Part model, mm, in its own coordinate system. Face numbers are marked on the shaded views. A direction names the side the tool comes from. Round coordinates to 2 decimals unless told otherwise and drop trailing zeros. Order: outer loops, then holes, each group sorted by start corner. A loop starts at its lowest first (then second) coordinate and runs counter-clockwise, first axis right, second up. Notation, with made-up numbers: (75, 62) -> (115, 62) arc R19 cw to (115, 73) -> close; hole circle Ø1 at (6, 87.5). An arc over 180 degrees is marked (long way). Answer as a JSON object with one key per item and string values. Group by question number.
```python
from build123d import *

# Parameters (mm, degrees)
SKETCH_1_W           = 20
SKETCH_1_H           = 20
EXTRUDE_1_DEPTH      = 120
SKETCH_2_W           = 10
SKETCH_2_H           = 20
CUT_EXTRUDE_1_DEPTH  = 120
CUT_EXTRUDE_2_DEPTH  = 120
SKETCH_4_R           = 3
CUT_EXTRUDE_3_DEPTH  = 2
SKETCH_8_W           = 19.6
SKETCH_8_H           = 0.2
SKETCH_8_W_2         = 0.2
SKETCH_8_H_2         = 19.6
CUT_EXTRUDE_6_DEPTH  = 15
SKETCH_9_W           = 10
SKETCH_9_H           = 20
CUT_EXTRUDE_7_DEPTH  = 20
SKETCH_10_W          = 19.6
SKETCH_10_H          = 19.6
EXTRUDE_2_DEPTH      = 15
CUT_EXTRUDE_8_DEPTH  = 20
CUT_EXTRUDE_9_DEPTH  = 20
SKETCH_13_W          = 55
SKETCH_13_H          = 20
SKETCH_13_W_2        = 18.82824967
CUT_EXTRUDE_10_DEPTH = 20
SKETCH_14_W          = 100
SKETCH_14_H          = 55
EXTRUDE_5_DEPTH      = 5
SKETCH_17_W          = 2
SKETCH_17_H          = 55
CUT_EXTRUDE_12_DEPTH = 1000
EXTRUDE_6_DEPTH      = 94
SKETCH_19_W          = 3
SKETCH_19_H          = 55
EXTRUDE_7_DEPTH      = 100


with BuildPart() as part:
    # 草图1 → 凸台-拉伸1 (new body)
    with BuildSketch(Plane.XY):
        with Locations((10, 10)):
            Rectangle(SKETCH_1_W, SKETCH_1_H)
    extrude(amount=EXTRUDE_1_DEPTH)

    # 草图2 → 切除-拉伸1 (cut)
    with BuildSketch(Plane(origin=(0, 20, 0), x_dir=(1, 0, 0), z_dir=(0, 1, 0))):
        with Locations((15, -10)):
            Rectangle(SKETCH_2_W, SKETCH_2_H)
    extrude(amount=-CUT_EXTRUDE_1_DEPTH, mode=Mode.SUBTRACT)

    # 草图3 → 切除-拉伸2 (cut)
    with BuildSketch(Plane(origin=(10, 0, 0), x_dir=(0, 0, -1), z_dir=(1, 0, 0))):
        with BuildLine():
            ThreePointArc((-8.45, 10), (-9.40684068, 11.432013275), (-11.096015511, 11.096015511))
            Line((-11.096015511, 11.096015511), (-8.903984489, 8.903984489))
            ThreePointArc((-8.903984489, 8.903984489), (-8.567986725, 9.40684068), (-8.45, 10))
        make_face()
        with BuildLine():
            Line((-8.903984489, 8.903984489), (-11.096015511, 11.096015511))
            ThreePointArc((-11.096015511, 11.096015511), (-11.096015511, 8.903984489), (-8.903984489, 8.903984489))
        make_face()
    extrude(amount=-CUT_EXTRUDE_2_DEPTH, mode=Mode.SUBTRACT)

    # 草图4 → 切除-拉伸3 (cut)
    with BuildSketch(Plane.ZY):
        with Locations((10, 10)):
            Circle(SKETCH_4_R)
    extrude(amount=-CUT_EXTRUDE_3_DEPTH, mode=Mode.SUBTRACT)

    # 草图8 → 切除-拉伸6 (cut)
    with BuildSketch(Plane.XY.offset(120)):
        with Locations((10, 19.9)):
            Rectangle(SKETCH_8_W, SKETCH_8_H)
        with Locations((0.1, 19.9)):
            Rectangle(SKETCH_8_W_2, SKETCH_8_H)
        with Locations((0.1, 10)):
            Rectangle(SKETCH_8_W_2, SKETCH_8_H_2)
        with Locations((19.9, 10)):
            Rectangle(SKETCH_8_W_2, SKETCH_8_H_2)
        with Locations((19.9, 0.1)):
            Rectangle(SKETCH_8_W_2, SKETCH_8_H)
        with Locations((10, 0.1)):
            Rectangle(SKETCH_8_W, SKETCH_8_H)
        with Locations((0.1, 0.1)):
            Rectangle(SKETCH_8_W_2, SKETCH_8_H)
        with Locations((19.9, 19.9)):
            Rectangle(SKETCH_8_W_2, SKETCH_8_H)
    extrude(amount=-CUT_EXTRUDE_6_DEPTH, mode=Mode.SUBTRACT)

    # 草图9 → 切除-拉伸7 (cut)
    with BuildSketch(Plane(origin=(0, 20, 0), x_dir=(1, 0, 0), z_dir=(0, 1, 0))):
        Polygon((0, 0), (0, -45), (20, -45), (20, -20), (10, -20), (10, 0), align=None)
        with Locations((15, -10)):
            Rectangle(SKETCH_9_W, SKETCH_9_H)
    extrude(amount=-CUT_EXTRUDE_7_DEPTH, mode=Mode.SUBTRACT)

    # 草图10 → 凸台-拉伸2 (add)
    with BuildSketch(Plane(origin=(0, 0, 45), x_dir=(-1, 0, 0), z_dir=(0, 0, -1))):
        with Locations((-10, 10)):
            Rectangle(SKETCH_10_W, SKETCH_10_H)
    extrude(amount=EXTRUDE_2_DEPTH)

    # 草图11 → 切除-拉伸8 (cut)
    with BuildSketch(Plane(origin=(0, 19.8, 0), x_dir=(1, 0, 0), z_dir=(0, 1, 0))):
        with BuildLine():
            ThreePointArc((11.547573501, -112.5), (10.487812185, -111.029569439), (8.757681845, -111.569855559))
            Line((8.757681845, -111.569855559), (11.237465157, -113.430144441))
            ThreePointArc((11.237465157, -113.430144441), (11.468004062, -112.990238683), (11.547573501, -112.5))
        make_face()
        with BuildLine():
            Line((11.237465157, -113.430144441), (8.757681845, -111.569855559))
            ThreePointArc((8.757681845, -111.569855559), (9.06742906, -113.739891656), (11.237465157, -113.430144441))
        make_face()
    extrude(amount=-CUT_EXTRUDE_8_DEPTH, mode=Mode.SUBTRACT)

    # 草图12 → 切除-拉伸9 (cut)
    with BuildSketch(Plane(origin=(0, 19.8, 0), x_dir=(1, 0, 0), z_dir=(0, 1, 0))):
        with BuildLine():
            ThreePointArc((11.55, -37.5), (10.490153037, -36.029540888), (8.76, -36.57))
            Line((8.76, -36.57), (11.24, -38.43))
            ThreePointArc((11.24, -38.43), (11.470459112, -37.990153037), (11.55, -37.5))
        make_face()
        with BuildLine():
            Line((11.24, -38.43), (8.76, -36.57))
            ThreePointArc((8.76, -36.57), (9.07, -38.74), (11.24, -38.43))
        make_face()
    extrude(amount=-CUT_EXTRUDE_9_DEPTH, mode=Mode.SUBTRACT)

    # 草图13 → 切除-拉伸10 (cut)
    with BuildSketch(Plane.ZY):
        with Locations((77.5, 10)):
            Rectangle(SKETCH_13_W, SKETCH_13_H)
        with Locations((114.414124835, 10)):
            Rectangle(SKETCH_13_W_2, SKETCH_13_H)
    extrude(amount=-CUT_EXTRUDE_10_DEPTH, mode=Mode.SUBTRACT)

    # 草图14 → 凸台-拉伸5 (add)
    with BuildSketch(Plane.XY.offset(50)):
        with Locations((10, 17.5)):
            Rectangle(SKETCH_14_W, SKETCH_14_H)
    extrude(amount=-EXTRUDE_5_DEPTH)

    # 草图17 → 切除-拉伸12 (cut)
    with BuildSketch(Plane.ZY.offset(40)):
        with Locations((49, 17.5)):
            Rectangle(SKETCH_17_W, SKETCH_17_H)
    extrude(amount=-CUT_EXTRUDE_12_DEPTH, mode=Mode.SUBTRACT)

    # 草图18 → 凸台-拉伸6 (add)
    with BuildSketch(Plane.XY.offset(48)):
        Polygon((-40, -10), (60, -10), (60, 45), (57, 45), (57, -7), (-37, -7), (-37, 45), (-40, 45), align=None)
    extrude(amount=EXTRUDE_6_DEPTH)

    # 草图19 → 凸台-拉伸7 (add)
    with BuildSketch(Plane(origin=(60, 0, 0), x_dir=(0, 0, -1), z_dir=(1, 0, 0))):
        with Locations((-143.5, 17.5)):
            Rectangle(SKETCH_19_W, SKETCH_19_H)
    extrude(amount=-EXTRUDE_7_DEPTH)


solid = part.part
```
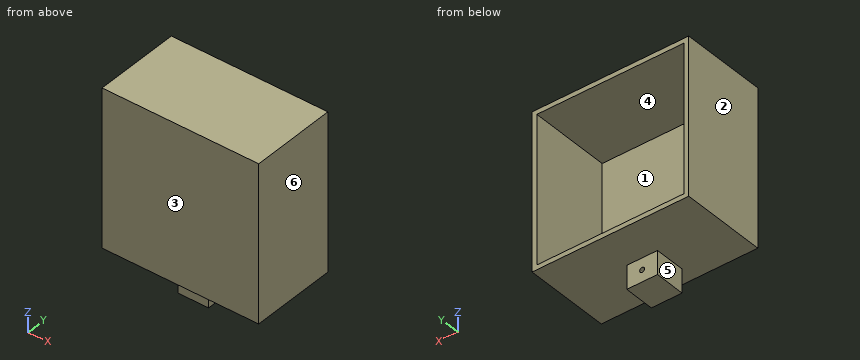
Q1. Band-saw the part on C-C (y = 35). List the corners of the cut face in (x, z).
Q2. Two-plate mould, pull along Y, no slides. Class the marked faces 1, 2 and 3: +Y half, -Y half, draft (parallel to the pull), parting line (faces both ways), or undercut.
Q3. Wall check: line 1 (Z direction, x = 10, y = 4.5); line 2 (Z direction, x = 5.5, y = -5); line 3 (X direction, y = 2, z = 82.5). Give the ranges that are in metal, low to high. Write a range as [from, to].
Q4. Band-saw the part on B-B (x = -26.5). List the corners of the cut face in (y, z).
Q5. Which spindle directions (+Z, -Z, +X, -X, +Y, -Y) get a long thin tool onto all of the face, cutting with end or side? Do the marked faces 4, 5 and 6. Say none if no direction does.
Q6. Band-saw the part on A-A (y = 8). List the corners of the cut face in (x, z).
Q7. Drop flat-ended pins along their axis: pin 1 Ø1.5 at (x, z) = (40.5, 115) entering from +Y; pin 2 Ø4.5 at (x, z) = (14, 34) entering from -Y; pin 3 Ø12 at (x, z) = (13.5, 34) entering from +Y. Give the stop position or say it passes through.
Q8. Band-saw the part on D-D (z = 110). List the corners of the cut face in (x, y), plus the area to 3 significant figures.
Completed:
{
 "1": {"outline": "(-40, 45) -> (60, 45) -> (60, 145) -> (-40, 145) -> close; hole (-37, 48) -> (57, 48) -> (57, 142) -> (-37, 142) -> close"},
 "2": {"face 1": "+Y half", "face 2": "draft", "face 3": "-Y half"},
 "3": {"line 1": "[30, 35.95], [39.05, 48], [142, 145]", "line 2": "[45, 48], [142, 145]", "line 3": "[-40, -37], [57, 60]"},
 "4": {"outline": "(-10, 45) -> (45, 45) -> (45, 48) -> (-7, 48) -> (-7, 142) -> (45, 142) -> (45, 145) -> (-10, 145) -> close"},
 "5": {"face 4": "+Y", "face 5": "-Z, -X, +Y, -Y", "face 6": "+Z, -Z, +X, +Y, -Y"},
 "6": {"outline": "(-40, 45) -> (0.2, 45) -> (0.2, 30) -> (19.8, 30) -> (19.8, 45) -> (60, 45) -> (60, 145) -> (-40, 145) -> close; hole (-37, 48) -> (57, 48) -> (57, 142) -> (-37, 142) -> close; hole circle Ø3.1 at (10, 37.5)"},
 "7": {"pin 1": "y = -7", "pin 2": "y = 0.2", "pin 3": "y = 19.8"},
 "8": {"outline": "(-40, -10) -> (60, -10) -> (60, 45) -> (57, 45) -> (57, -7) -> (-37, -7) -> (-37, 45) -> (-40, 45) -> close", "area": "612 mm2"}
}
